Could you check a few things on this model? Use its own coordinates, in mm. A direction names the side the tool comes from. Give positions to 0.01 mm unless a question says otherwise; leave off trailing zeros. Order: outer loops, then holes, each group sorted by start corner. A loop starts at its lowest first (then second) coordinate and runs counter-clockwise, first axis right, second up.
(1) Imagine slicing it at D-D, the plane x = -13. Write out the boundary of the cut face in (y, z).
(2) Imagine slicing it at C-C, the plane z = 4.4. State how many separate pieces and enclosed holes the cut face has, then the cut area to 3 significant figures.
(3) Imagine slicing it at B-B, the plane y = 31.5. Write out the boundary of the cut face in (x, z).
(4) Will these pins go through, and if not, where does the flat tip stop? pin 1 (1.8 mm diameter, centred on x = -90.5, z = 3.5, fed in from +Y); pin 2 (3 mm diameter, centred on x = -41.5, z = 4, fed in from +Y); pin 3 (2 mm diameter, centred on x = -43.5, z = 4, fed in from +Y); pin 4 (8 mm diameter, centred on x = -22.5, y = -1.5, fed in from +Z).
(5) If we mould it in two halves opening along Y, with no side actions, what happens to faces 1 (the flat face through (21, -25, 6)), 2 (the flat face through (-90, -41.5, 3)), 3 (the flat face through (-95, 18.5, 3))? For each: released by +Y, released by -Y, zero draft, split by the parting line, or undercut.
(6) Imagine slicing it at A-A, the plane x = 33.5. Write out the boundary of the cut face in (y, z).
(7) If I drill on probe 1 along X at (y, z) = (-28, 0.5); probe 2 along X at (y, z) = (-10.5, 0.65); probe 3 along Y at (x, z) = (24, 0.95), over which ranges is the centre line in solid material (lowest first)?
(8) On a 3-axis mill with a long thin cutter (end or side, diameter ignored), from which of +Z, -Z, +X, -X, +Y, -Y can I reach the whole of each face in a straight line? I mean faces 4 (the flat face through (-74, -6.5, 3)), 5 (the flat face through (103, 32, 3)), 6 (the flat face through (38, 93.5, 3)), 7 (the flat face through (79, -32, 3)), 8 (the flat face through (21, -25, 0)). Say none if no direction works.
Solid Edge part; units mm, degrees
sketch "Sketch1" plane through (0, 0, 0) normal (0, 0, 1) x (1, 0, 0)
  line L0 (-87, -21.5) -> (-93, -21.5)
  line L1 (-93, -21.5) -> (-93, -41.5)
  line L2 (-93, -41.5) -> (-87, -41.5)
  line L3 (-87, -41.5) -> (-87, -21.5)
  line L4 (79, -21.5) -> (73, -21.5)
  line L5 (73, -21.5) -> (73, -41.5)
  line L6 (73, -41.5) -> (79, -41.5)
  line L7 (79, -41.5) -> (79, -21.5)
  line L8 (81.75, 23.5) -> (94.25, 23.5)
  line L9 (94.25, 23.5) -> (94.25, 46.5)
  line L10 (94.25, 46.5) -> (81.75, 46.5)
  line L11 (81.75, 46.5) -> (81.75, 23.5)
  line L12 (103, 93.5) -> (103, 123.5)
  line L13 (103, 123.5) -> (3, 123.5)
  line L14 (3, 123.5) -> (3, 93.5)
  line L15 (3, 93.5) -> (73, 93.5)
  line L16 (73, 56.5) -> (73, 93.5)
  line L17 (73, 56.5) -> (73, -6.5)
  line L18 (73, -6.5) -> (48, -6.5)
  line L19 (48, -6.5) -> (48, -12.5)
  line L20 (48, -12.5) -> (28, -12.5)
  line L21 (28, -12.5) -> (28, -6.5)
  line L22 (28, -6.5) -> (-42, -6.5)
  line L23 (-42, -6.5) -> (-42, -12.5)
  line L24 (-42, -12.5) -> (-62, -12.5)
  line L25 (-62, -12.5) -> (-62, -6.5)
  line L26 (-62, -6.5) -> (-87, -6.5)
  line L27 (-87, -6.5) -> (-87, 18.5)
  line L28 (-87, 18.5) -> (-103, 18.5)
  line L29 (-103, 18.5) -> (-103, -56.5)
  line L30 (-103, -56.5) -> (103, -56.5)
  line L31 (103, -56.5) -> (103, 56.5)
  line L32 (103, 93.5) -> (103, 56.5)
  dimension "D1" = 103
  dimension "D2" = 73
  dimension "D3" = 87
  dimension "D4" = 93
  dimension "D5" = 79
  dimension "D6" = 73
  dimension "D7" = 79
  dimension "D8" = 42
  dimension "D9" = 48
  dimension "D10" = 48
  dimension "D11" = 42
  dimension "D12" = 28
  dimension "D13" = 103
  dimension "D14" = 87
  dimension "D15" = 103
  dimension "D16" = 62
  dimension "D17" = 94.25
  dimension "D18" = 81.75
  dimension "D19" = 103
  dimension "D20" = 103
extrude "Protrusion1" add sketch "Sketch1" along normal blind 6
Answer block:
1. outline: (-56.5, 0) - (-6.5, 0) - (-6.5, 6) - (-56.5, 6) - close
2. separate pieces: 1
2. enclosed holes: 3
2. area: 15,900 mm2
3. outline: (73, 0) - (81.75, 0) - (81.75, 6) - (73, 6) - close; (94.25, 0) - (103, 0) - (103, 6) - (94.25, 6) - close
4. pin 1: stops at y = 18.5
4. pin 2: stops at y = -6.5
4. pin 3: stops at y = -12.5
4. pin 4: passes through
5. face 1: zero draft
5. face 2: undercut
5. face 3: released by +Y
6. outline: (-56.5, 0) - (-12.5, 0) - (-12.5, 6) - (-56.5, 6) - close; (93.5, 0) - (123.5, 0) - (123.5, 6) - (93.5, 6) - close
7. probe 1: x = -103 to -93, -87 to 73, 79 to 103
7. probe 2: x = -103 to -62, -42 to 28, 48 to 103
7. probe 3: y = -56.5 to -6.5, 93.5 to 123.5
8. face 4: +Z, -Z, +Y
8. face 5: +Z, -Z, +X, +Y, -Y
8. face 6: +Z, -Z, -X
8. face 7: +Z, -Z
8. face 8: -Z, +X, -X, +Y, -Y
